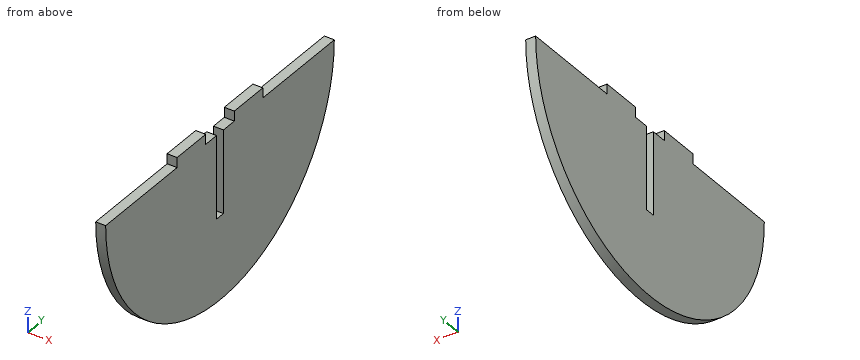
```python
from build123d import *

# Parameters (mm, degrees)
F1_DEPTH = 3.048


with BuildPart() as f1:
    # F0 (on Right) → F1 (new body)
    with BuildSketch(Plane.YZ):
        with BuildLine():
            Line((-19.05, 50.8), (-50.8, 50.8))
            ThreePointArc((-50.8, 50.8), (0, 0), (50.8, 50.8))
            Line((50.8, 50.8), (19.05, 50.8))
            Line((19.05, 50.8), (19.05, 53.848))
            Line((19.05, 53.848), (6.35, 53.848))
            Line((6.35, 53.848), (6.35, 50.8))
            Line((6.35, 50.8), (1.524, 50.8))
            Line((1.524, 50.8), (1.524, 25.4))
            Line((1.524, 25.4), (-1.524, 25.4))
            Line((-1.524, 25.4), (-1.524, 50.8))
            Line((-1.524, 50.8), (-6.35, 50.8))
            Line((-6.35, 50.8), (-6.35, 53.848))
            Line((-6.35, 53.848), (-19.05, 53.848))
            Line((-19.05, 53.848), (-19.05, 50.8))
        make_face()
    extrude(amount=F1_DEPTH)


solid = f1.part
```
Geometry check sheet. Reference: the model listing, model coordinates, mm. Give positions to 0.01 mm unless a question says otherwise; leave off trailing zeros. Write each loop counter-clockwise with the first axis right and the second up, starting at its lowest first coordinate (ties: lowest second). Pieces come first, ordered by that corner, then holes.
1) Material ranges on L1, parallel to Y at x = 0.6, z = 51.5; L2, parallel to Y at x = 2.7, z = 44; L3, parallel to Z at x = 2.6, y = -22, recorded low to high.
2) Section check A-A, the plane z = 30.5. Record the boundary of the cut face in (x, y), and give its area (3 significant figures).
3) Section check D-D, the plane z = 47. Record the boundary of the cut face in (x, y).
4) Section check B-B, the plane x = 1.1. Record the boundary of the cut face in (y, z).
5) Gauge pin test, flat ends, axial feed: pin 1 (3 mm diameter, centred on y = -1.5, z = 7.5, fed in from -X); pin 2 (1.5 mm diameter, centred on x = 1, z = 44, fed in from +Y); pin 3 (1.5 mm diameter, centred on x = 2, z = 52.5, fed in from +Y); pin 4 (0.9 mm diameter, centred on x = 1, z = 40, fed in from -Y). Record the tip position at first contact, or that the pin passes through.
6) Section check C-C, the plane y = -14. Record the boundary of the cut face in (x, z), and give its area (3 significant figures).
Computed:
1. L1: y = -19.05 to -6.35, 6.35 to 19.05
1. L2: y = -50.34 to -1.52, 1.52 to 50.34
1. L3: z = 5.01 to 50.8
2. outline: (0, -46.57) - (3.05, -46.57) - (3.05, -1.52) - (0, -1.52) - close; (0, 1.52) - (3.05, 1.52) - (3.05, 46.57) - (0, 46.57) - close
2. area: 275 mm2
3. outline: (0, -50.66) - (3.05, -50.66) - (3.05, -1.52) - (0, -1.52) - close; (0, 1.52) - (3.05, 1.52) - (3.05, 50.66) - (0, 50.66) - close
4. outline: (-50.8, 50.8) arc R50.8 ccw to (50.8, 50.8) - (19.05, 50.8) - (19.05, 53.85) - (6.35, 53.85) - (6.35, 50.8) - (1.52, 50.8) - (1.52, 25.4) - (-1.52, 25.4) - (-1.52, 50.8) - (-6.35, 50.8) - (-6.35, 53.85) - (-19.05, 53.85) - (-19.05, 50.8) - close
5. pin 1: stops at x = 0
5. pin 2: stops at y = 50.44
5. pin 3: stops at y = 19.05
5. pin 4: stops at y = -49.73
6. outline: (0, 1.97) - (3.05, 1.97) - (3.05, 53.85) - (0, 53.85) - close
6. area: 158 mm2
